Design review of the part built by this model. Coordinates are the model's own, in mm. Coordinates: 2 decimals unless noted, no trailing zeros. Loops run counter-clockwise (first coordinate to the right, second up) from the corner with the lowest first, then second, coordinate; pieces in that order, holes last. Notation, with made-up numbers: (29.5, 9.25) -> (78.5, 9.25) arc R6 cw to (78.5, 13.25) -> close; hole circle Ø7 at (67.5, 80). An arc over 180 degrees is marked (long way). One line per item, written item: value. Start each with the question number.
1. Add section A-A on z = 0. Write out the cut boundary in (x, y), plus the area to 3 significant figures.
2. Add section C-C on x = -34. Write out the cut boundary in (y, z), plus the area to 3 significant figures.
3. For probe 1 along X at (y, z) = (0.6, 50); probe 2 along Z at (x, y) = (34, 1.05); probe 3 along X at (y, z) = (0.4, 0), list the stretches that pass through material, from the lowest coordinate up.
4. Insertion check: pin 1 (4.5 mm diameter, centred on x = 0, z = 0, fed in from -Y). The pin has a flat end and moves straight along its axis. Give the tip position at first contact, or say it passes through.
5. Add section B-B on x = 0. Write out the cut boundary in (y, z).
6. Draft analysis for pull direction X (two halves, no side actions). For faces 1 (the cylindrical face through (0.77, 0.99, 2.43)), 2 (the flat face through (12, 0, -1)), 3 (the cylindrical face through (34.325, 0.986, -48.536)), state which applies: pulls with the +X half, pulls with the -X half, needs draft (parallel to the pull), parting line crosses it, or undercut.
```python
from build123d import *

# Parameters (mm, degrees)
SKETCH1_W             = 115
SKETCH1_H             = 115
SKETCH1_R             = 2.55
BOSS_EXTRUDE1_DEPTH   = 2
F_3_0MM_DOWEL_HOLE1_D = 3


with BuildPart() as part:
    # Sketch1 → Boss-Extrude1 (new body)
    with BuildSketch(Plane(origin=(0, 0, 0), x_dir=(1, 0, 0), z_dir=(0, 1, 0))):
        Rectangle(SKETCH1_W, SKETCH1_H)
        with Locations(Location((0, 0, 0), (0, 0, 270))):
            Circle(SKETCH1_R, mode=Mode.SUBTRACT)
    extrude(amount=BOSS_EXTRUDE1_DEPTH)

    # Ø3.0mm Dowel Hole1 (through all)
    with Locations(Plane(origin=(0, 2, 0), x_dir=(1, 0, 0), z_dir=(0, 1, 0))):
        with Locations((-34, 50), (34, 50), (34, -50), (-34, -50)):
            Hole(F_3_0MM_DOWEL_HOLE1_D / 2)


solid = part.part
```
Worked answers:
1. outline: (-57.5, 0) -> (-2.55, 0) -> (-2.55, 2) -> (-57.5, 2) -> close; (2.55, 0) -> (57.5, 0) -> (57.5, 2) -> (2.55, 2) -> close
1. area: 220 mm²
2. outline: (0, -57.5) -> (2, -57.5) -> (2, -51.5) -> (0, -51.5) -> close; (0, -48.5) -> (2, -48.5) -> (2, 48.5) -> (0, 48.5) -> close; (0, 51.5) -> (2, 51.5) -> (2, 57.5) -> (0, 57.5) -> close
2. area: 218 mm²
3. probe 1: x = -57.5 to -35.5, -32.5 to 32.5, 35.5 to 57.5
3. probe 2: z = -57.5 to -51.5, -48.5 to 48.5, 51.5 to 57.5
3. probe 3: x = -57.5 to -2.55, 2.55 to 57.5
4. pin 1: passes through
5. outline: (0, -57.5) -> (2, -57.5) -> (2, -2.55) -> (0, -2.55) -> close; (0, 2.55) -> (2, 2.55) -> (2, 57.5) -> (0, 57.5) -> close
6. face 1: undercut
6. face 2: needs draft
6. face 3: undercut
